Check sheet for the modelled part. Datum: model origin and axes. Units: mm. Round coordinates to 2 decimals unless told otherwise and drop trailing zeros. Write each loop counter-clockwise with the first axis right and the second up, starting at its lowest first coordinate (ties: lowest second). Pieces come first, ordered by that corner, then holes. Notation, with made-up numbers: (-31.5, 60.5) -> (-25.5, 60.5) arc R30 cw to (-25.5, 97.5) -> close; hole circle Ø11 at (9, 66). An arc over 180 degrees is marked (long way). Write item = value, one per line.
from build123d import *


with BuildPart() as part:
    # Sketch1 → Revolve1 (revolve)
    with BuildSketch(Plane(origin=(0, 0, 0), x_dir=(0, 0, -1), z_dir=(1, 0, 0)), mode=Mode.PRIVATE) as revolve1_sk:
        with BuildLine():
            Line((0, 52.5), (1.5, 52))
            Line((1.5, 52), (1.5, 49.5))
            Line((1.5, 49.5), (0.9, 49.5))
            ThreePointArc((0.9, 49.5), (0, 49.8), (-0.9, 49.5))
            Line((-0.9, 49.5), (-1.5, 49.5))
            Line((-1.5, 49.5), (-1.5, 52))
            Line((-1.5, 52), (0, 52.5))
        make_face()
    revolve(revolve1_sk.sketch.rotate(Axis((0, 0, 0), (0, 0, -1)), 90), axis=Axis((0, 0, 0), (0, 0, -1)))


solid = part.part
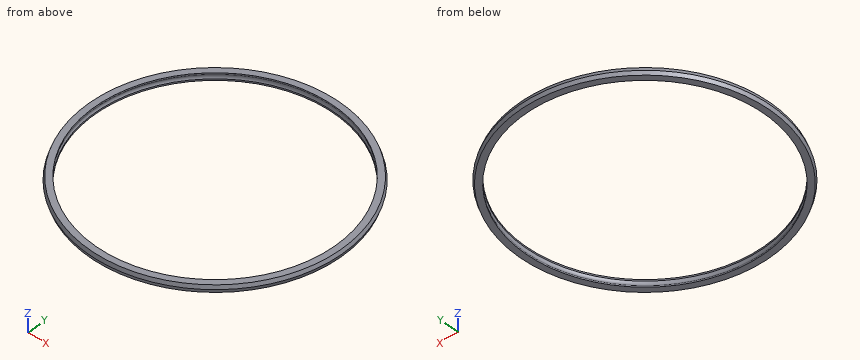
(1) Material ranges on L1, parallel to Y at x = 0, z = -1.4; L2, parallel to Y at x = -2, z = 0.8; L3, parallel to X at y = 31.5, z = -0.25, recorded low to high. Write a range as [from, to].
Worked answers:
L1 = [-52.03, -49.5], [49.5, 52.03]
L2 = [-52.2, -49.53], [49.53, 52.2]
L3 = [-41.9, -38.54], [38.54, 41.9]
(2) Go/stop test with flat-tipped pins: P1, Ø1, axis at y = 10.5, z = 0.5, coming from the +X side; P2, Ø1, axis at x = -34, z = 0.5, coming from the -Y side. Record where each tip stops, or that it passes through.
Worked answers:
P1 = 51.47
P2 = -40.26
(3) Sectioned sample at A-A on y = 0. Enter the section's corners in (x, z), then the cut area to 3 significant figures.
Worked answers:
outline = (-52.5, 0) -> (-52, -1.5) -> (-49.5, -1.5) -> (-49.5, -0.9) arc R1.5 cw to (-49.5, 0.9) -> (-49.5, 1.5) -> (-52, 1.5) -> close; (49.5, -1.5) -> (52, -1.5) -> (52.5, 0) -> (52, 1.5) -> (49.5, 1.5) -> (49.5, 0.9) arc R1.5 cw to (49.5, -0.9) -> close
area = 15.8 mm²
